```python
from build123d import *

# Parameters (mm, degrees)
BOSS_EXTRUDE1_DEPTH = 425


with BuildPart() as part:
    # Sketch1 → Boss-Extrude1 (new body)
    with BuildSketch(Plane(origin=(0, 0, 0), x_dir=(1, 0, 0), z_dir=(0, 1, 0))):
        with BuildLine():
            Line((0, 3.65), (0, 11.726074497))
            ThreePointArc((0, 11.726074497), (0.973229377, 13.937906507), (3.261467228, 14.714658591))
            Line((3.261467228, 14.714658591), (27.261467228, 12.614930666))
            ThreePointArc((27.261467228, 12.614930666), (29.21183201, 11.653117195), (30, 9.626346572))
            Line((30, 9.626346572), (30, 4.25))
            ThreePointArc((30, 4.25), (29.956066017, 4.143933983), (29.85, 4.1))
            Line((29.85, 4.1), (28.65, 4.1))
            ThreePointArc((28.65, 4.1), (28.543933983, 4.143933983), (28.5, 4.25))
            Line((28.5, 4.25), (28.5, 9.626346572))
            ThreePointArc((28.5, 9.626346572), (28.105916005, 10.639731884), (27.130733614, 11.120638619))
            Line((27.130733614, 11.120638619), (22.463073361, 11.529005977))
            ThreePointArc((22.463073361, 11.529005977), (22.348661469, 11.490168372), (22.3, 11.379576772))
            Line((22.3, 11.379576772), (22.3, -11.379576772))
            ThreePointArc((22.3, -11.379576772), (22.348661469, -11.490168372), (22.463073361, -11.529005977))
            Line((22.463073361, -11.529005977), (27.130733614, -11.120638619))
            ThreePointArc((27.130733614, -11.120638619), (28.105916005, -10.639731884), (28.5, -9.626346572))
            Line((28.5, -9.626346572), (28.5, -4.25))
            ThreePointArc((28.5, -4.25), (28.543933983, -4.143933983), (28.65, -4.1))
            Line((28.65, -4.1), (29.85, -4.1))
            ThreePointArc((29.85, -4.1), (29.956066017, -4.143933983), (30, -4.25))
            Line((30, -4.25), (30, -9.626346572))
            ThreePointArc((30, -9.626346572), (29.21183201, -11.653117195), (27.261467228, -12.614930666))
            Line((27.261467228, -12.614930666), (3.261467228, -14.714658591))
            ThreePointArc((3.261467228, -14.714658591), (0.973229377, -13.937906507), (0, -11.726074497))
            Line((0, -11.726074497), (0, -3.65))
            ThreePointArc((0, -3.65), (-0.193830765, -3.336772973), (-0.560635258, -3.370477571))
            Line((-0.560635258, -3.370477571), (-1.241594271, -3.883616994))
            ThreePointArc((-1.241594271, -3.883616994), (-1.321364591, -3.936115739), (-1.407159256, -3.978052566))
            ThreePointArc((-1.407159256, -3.978052566), (-1.474647279, -4.03329008), (-1.5, -4.116735006))
            Line((-1.5, -4.116735006), (-1.5, -4.895206856))
            ThreePointArc((-1.5, -4.895206856), (-1.531192993, -4.986775929), (-1.611798603, -5.040260823))
            ThreePointArc((-1.611798603, -5.040260823), (-4.945770747, -4.732123456), (-7.298777867, -2.350175433))
            ThreePointArc((-7.298777867, -2.350175433), (-7.305313905, -2.242111424), (-7.237408738, -2.157793941))
            Line((-7.237408738, -2.157793941), (-6.681980515, -1.837117307))
            ThreePointArc((-6.681980515, -1.837117307), (-6.186662348, -1.74635024), (-5.745584412, -1.989309088))
            ThreePointArc((-5.745584412, -1.989309088), (-3.556386599, -2.999470045), (-1.330769231, -2.072302553))
            ThreePointArc((-1.330769231, -2.072302553), (-1.240582163, -2.011981832), (-1.133333333, -1.995550606))
            ThreePointArc((-1.133333333, -1.995550606), (1, 0), (-1.133333333, 1.995550606))
            ThreePointArc((-1.133333333, 1.995550606), (-1.240582163, 2.011981832), (-1.330769231, 2.072302553))
            ThreePointArc((-1.330769231, 2.072302553), (-3.556386599, 2.999470045), (-5.745584412, 1.989309088))
            ThreePointArc((-5.745584412, 1.989309088), (-6.186662348, 1.74635024), (-6.681980515, 1.837117307))
            Line((-6.681980515, 1.837117307), (-7.237408738, 2.157793941))
            ThreePointArc((-7.237408738, 2.157793941), (-7.305313905, 2.242111424), (-7.298777867, 2.350175433))
            ThreePointArc((-7.298777867, 2.350175433), (-4.945770747, 4.732123456), (-1.611798603, 5.040260823))
            ThreePointArc((-1.611798603, 5.040260823), (-1.531192993, 4.986775929), (-1.5, 4.895206856))
            Line((-1.5, 4.895206856), (-1.5, 4.116735006))
            ThreePointArc((-1.5, 4.116735006), (-1.474647279, 4.03329008), (-1.407159256, 3.978052566))
            ThreePointArc((-1.407159256, 3.978052566), (-1.321364591, 3.936115739), (-1.241594271, 3.883616994))
            Line((-1.241594271, 3.883616994), (-0.560635258, 3.370477571))
            ThreePointArc((-0.560635258, 3.370477571), (-0.193830765, 3.336772973), (0, 3.65))
        make_face()
        with BuildLine():
            Line((1.5, 3.75), (1.5, 11.726074497))
            ThreePointArc((1.5, 11.726074497), (1.986614689, 12.831990502), (3.130733614, 13.220366544))
            Line((3.130733614, 13.220366544), (20.663073361, 11.686485571))
            ThreePointArc((20.663073361, 11.686485571), (20.760591601, 11.638394897), (20.8, 11.537056366))
            Line((20.8, 11.537056366), (20.8, 6.268971207))
            ThreePointArc((20.8, 6.268971207), (20.373749385, 5.592446015), (19.579503106, 5.684905567))
            ThreePointArc((19.579503106, 5.684905567), (12.478865683, 6.850830735), (7.827850799, 1.360248447))
            ThreePointArc((7.827850799, 1.360248447), (7.569361706, 0.92236964), (7.090986155, 0.75))
            Line((7.090986155, 0.75), (4.5, 0.75))
            ThreePointArc((4.5, 0.75), (2.378679656, 1.628679656), (1.5, 3.75))
        make_face(mode=Mode.SUBTRACT)
        with BuildLine():
            Line((3.130733614, -13.220366544), (20.663073361, -11.686485571))
            ThreePointArc((20.663073361, -11.686485571), (20.760591601, -11.638394897), (20.8, -11.537056366))
            Line((20.8, -11.537056366), (20.8, -6.268971207))
            ThreePointArc((20.8, -6.268971207), (20.373749385, -5.592446015), (19.579503106, -5.684905567))
            ThreePointArc((19.579503106, -5.684905567), (12.478865683, -6.850830735), (7.827850799, -1.360248447))
            ThreePointArc((7.827850799, -1.360248447), (7.569361706, -0.92236964), (7.090986155, -0.75))
            Line((7.090986155, -0.75), (4.5, -0.75))
            ThreePointArc((4.5, -0.75), (2.378679656, -1.628679656), (1.5, -3.75))
            Line((1.5, -3.75), (1.5, -11.726074497))
            ThreePointArc((1.5, -11.726074497), (1.986614689, -12.831990502), (3.130733614, -13.220366544))
        make_face(mode=Mode.SUBTRACT)
        with BuildLine():
            Line((11.95237619, 4.744680085), (12.554594319, 4.142461956))
            ThreePointArc((12.554594319, 4.142461956), (12.93723035, 3.937478186), (13.369341573, 3.978813026))
            ThreePointArc((13.369341573, 3.978813026), (15, 4.3), (16.630658427, 3.978813026))
            ThreePointArc((16.630658427, 3.978813026), (17.06276965, 3.937478186), (17.445405681, 4.142461956))
            Line((17.445405681, 4.142461956), (18.04762381, 4.744680085))
            ThreePointArc((18.04762381, 4.744680085), (18.171115834, 4.802453455), (18.302939637, 4.767660826))
            ThreePointArc((18.302939637, 4.767660826), (19.101219331, 4.101219331), (19.767660826, 3.302939637))
            ThreePointArc((19.767660826, 3.302939637), (19.802453455, 3.171115834), (19.744680085, 3.04762381))
            Line((19.744680085, 3.04762381), (19.142461956, 2.445405681))
            ThreePointArc((19.142461956, 2.445405681), (18.937478186, 2.06276965), (18.978813026, 1.630658427))
            ThreePointArc((18.978813026, 1.630658427), (19.3, 0), (18.978813026, -1.630658427))
            ThreePointArc((18.978813026, -1.630658427), (18.937478186, -2.06276965), (19.142461956, -2.445405681))
            Line((19.142461956, -2.445405681), (19.744680085, -3.04762381))
            ThreePointArc((19.744680085, -3.04762381), (19.802453455, -3.171115834), (19.767660826, -3.302939637))
            ThreePointArc((19.767660826, -3.302939637), (19.101219331, -4.101219331), (18.302939637, -4.767660826))
            ThreePointArc((18.302939637, -4.767660826), (18.171115834, -4.802453455), (18.04762381, -4.744680085))
            Line((18.04762381, -4.744680085), (17.445405681, -4.142461956))
            ThreePointArc((17.445405681, -4.142461956), (17.06276965, -3.937478186), (16.630658427, -3.978813026))
            ThreePointArc((16.630658427, -3.978813026), (15, -4.3), (13.369341573, -3.978813026))
            ThreePointArc((13.369341573, -3.978813026), (12.93723035, -3.937478186), (12.554594319, -4.142461956))
            Line((12.554594319, -4.142461956), (11.95237619, -4.744680085))
            ThreePointArc((11.95237619, -4.744680085), (11.828884166, -4.802453455), (11.697060363, -4.767660826))
            ThreePointArc((11.697060363, -4.767660826), (10.898780669, -4.101219331), (10.232339174, -3.302939637))
            ThreePointArc((10.232339174, -3.302939637), (10.197546545, -3.171115834), (10.255319915, -3.04762381))
            Line((10.255319915, -3.04762381), (10.857538044, -2.445405681))
            ThreePointArc((10.857538044, -2.445405681), (11.062521814, -2.06276965), (11.021186974, -1.630658427))
            ThreePointArc((11.021186974, -1.630658427), (10.7, 0), (11.021186974, 1.630658427))
            ThreePointArc((11.021186974, 1.630658427), (11.062521814, 2.06276965), (10.857538044, 2.445405681))
            Line((10.857538044, 2.445405681), (10.255319915, 3.04762381))
            ThreePointArc((10.255319915, 3.04762381), (10.197546545, 3.171115834), (10.232339174, 3.302939637))
            ThreePointArc((10.232339174, 3.302939637), (10.898780669, 4.101219331), (11.697060363, 4.767660826))
            ThreePointArc((11.697060363, 4.767660826), (11.828884166, 4.802453455), (11.95237619, 4.744680085))
        make_face(mode=Mode.SUBTRACT)
    extrude(amount=BOSS_EXTRUDE1_DEPTH)


solid = part.part
```
Here's how the part is built. I have some questions about the finished solid (model axes, mm). A direction names the side the tool comes from. Give positions to 0.01 mm unless a question says otherwise; leave off trailing zeros. Use CSV: the item, a comma, the result in double quotes. Start each with the question number.
Item 1: On a 3-axis mill with a long thin cutter (end or side, diameter ignored), from which of +Z, -Z, +X, -X, +Y, -Y can I reach the whole of each face in a straight line? I mean faces 5 (the flat face through (0, 210, 8)), 6 (the flat face through (0, 210, -8)), 7 (the flat face through (11.774, 209.525, 12.464)), 8 (the flat face through (15.43, 209.52, 13.65)). Say none if no direction works.
Item 2: I'm going to push flat-ended pins straight in: P1, Ø1.6, axis at y = 210.5, z = 8, coming from the -X side; P2, Ø1.3, axis at x = 6.5, y = 255, coming from the +Z side; P3, Ø6, axis at x = 9.5, z = 9.5, coming from the -Y side; P4, Ø12, axis at x = 13, y = 44.5, coming from the -Z side. Where does each tip first touch, or does it pass through?
Item 3: If I drill on probe 1 along X at (y, z) = (40, -9); probe 2 along X at (y, z) = (182.5, 6.5); probe 3 along Z at (x, y) = (-1, 309), over which ranges is the centre line in solid material (lowest first)? Write a range as [from, to].
Item 4: Suppose I cut it at A-A (y = 63). Give the number of separate pieces and of enclosed holes in the cut face, and give its area (3 significant figures).
Item 5: Thinking about a two-plate mould opening in Z: for faces 1 (the flat face through (10, 425, 1)), 2 (the cylindrical face through (12.578, 209.525, 6.886)), 3 (the flat face through (15.09, 209.52, -13.68)), 4 (the cylindrical face through (12.578, 209.525, -6.886)), which applies, pulls with the +Z half, pulls with the -Z half, needs draft (parallel to the pull), parting line crosses it, or undercut?
Answer block:
1,face 5,"+Z, +Y, -Y"
1,face 6,"-Z, +Y, -Y"
1,face 7,"+Y, -Y"
1,face 8,"+Z, +X, +Y, -Y"
2,P1,"stops at x = 0"
2,P2,"stops at z = 14.49"
2,P3,"passes through"
2,P4,"stops at z = -14.39"
3,probe 1,"x = [0, 1.5], [20.8, 22.3], [28.5, 30]"
3,probe 2,"x = [0, 1.5], [11.68, 18.32], [20.8, 22.3], [28.5, 30]"
3,probe 3,"z = [-3.7, -2], [2, 3.7]"
4,separate pieces,"1"
4,enclosed holes,"3"
4,area,"307 mm^2"
5,face 1,"needs draft"
5,face 2,"undercut"
5,face 3,"pulls with the -Z half"
5,face 4,"undercut"
